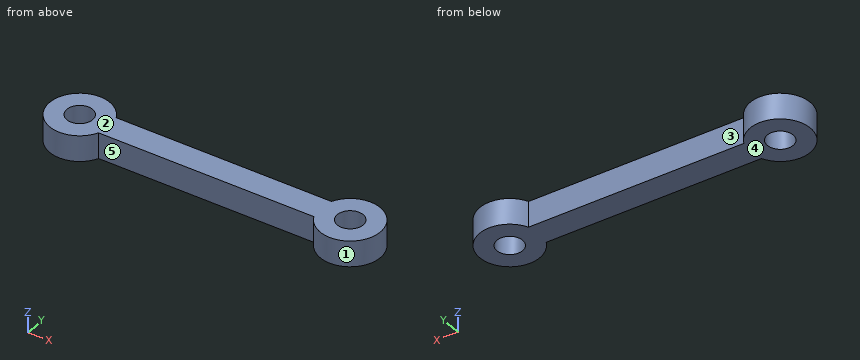
Autodesk Fusion 360 part; units mm, degrees
sketch "Sketch1" plane through (0, 0, 0) normal (0, 0, 1) x (1, 0, 0)
  circle A0 centre (-30.1129, -14.4636) radius 3.5
  circle A1 centre (-30.1129, -14.4636) radius 1.5
  line L0 (-30.1129, -14.4636) -> (0.8871, -14.4636)
  line L1 (-14.6129, -4.9636) -> (-14.6129, -23.9636) construction
  circle A2 centre (0.8871, -14.4636) radius 3.5
  circle A3 centre (0.8871, -14.4636) radius 1.5
  line L2 (-26.9506, -12.9636) -> (-2.2752, -12.9636)
  line L3 (-26.9506, -15.9636) -> (-2.2752, -15.9636)
  point P0 (0.8871, -14.4636)
  dimension "d1" = 7
  dimension "d2" = 3
  dimension "d3" = 31
  dimension "d4" = 1.5
extrude "Extrude1" add sketch "Sketch1" along normal blind 3
Design review of the part built by this model. Coordinates are the model's own, in mm. Face numbers are marked on the shaded views. A direction names the side the tool comes from. Coordinates: 2 decimals unless noted, no trailing zeros. Loops run counter-clockwise (first coordinate to the right, second up) from the corner with the lowest first, then second, coordinate; pieces in that order, holes last. Notation, with made-up numbers: (11, 40.25) -> (42, 40.25) arc R19 ccw to (42, 68.25) -> close; hole circle Ø8 at (10, -14.75). An arc over 180 degrees is marked (long way). Answer as a JSON object with one key per item and string values.
Q1. Take a section at C-C on z = 1.15. Give the boundary of the cut face in (x, y), plus the area to 3 significant figures.
Answer block:
{"outline": "(-26.95, -15.96) -> (-2.28, -15.96) arc R3.5 ccw (long way) to (-2.28, -12.96) -> (-26.95, -12.96) arc R3.5 ccw (long way) to start; hole circle Ø3 at (-30.11, -14.46); hole circle Ø3 at (0.89, -14.46)", "area": "135 mm^2"}
Q2. Take a section at D-D on x = -14. Give the boundary of the cut face in (y, z).
Answer block:
{"outline": "(-15.96, 0) -> (-12.96, 0) -> (-12.96, 3) -> (-15.96, 3) -> close"}
Q3. To check wall thickness, follow L1, parallel to X at y = -15, z = 0.75; L2, parallel to X at y = -14.75, z = 1.8; L3, parallel to Y at x = -13, z = 1.3. State the ranges of each line that lie inside material, in increasing order.
Answer block:
{"L1": "x = -33.57 to -31.51, -28.71 to -0.51, 2.29 to 4.35", "L2": "x = -33.6 to -31.59, -28.64 to -0.59, 2.36 to 4.38", "L3": "y = -15.96 to -12.96"}
Q4. The part is to be moulded in two halves that separate along X. For the marked faces 1 and 2, say which applies: +X half, -X half, draft (parallel to the pull), parting line (faces both ways), or undercut.
Answer block:
{"face 1": "undercut", "face 2": "draft"}
Q5. Tool access review of the marked faces 3, 4 and 5: name each direction out of +Z, -Z, +X, -X, +Y, -Y from which nothing blocks a thin tool from reaching the whole face with its end or side.
Answer block:
{"face 3": "+Z, -Z, +Y", "face 4": "-Z, +X, -X, +Y, -Y", "face 5": "+Z, -Z, -Y"}
Q6. Take a section at A-A on y = -17. Give the boundary of the cut face in (x, z).
Answer block:
{"outline": "(-32.52, 0) -> (-27.7, 0) -> (-27.7, 3) -> (-32.52, 3) -> close; (-1.52, 0) -> (3.3, 0) -> (3.3, 3) -> (-1.52, 3) -> close"}
Q7. Clearance check with a flat-ended pin moving along its axis: pin 1 Ø1.5 at (y, z) = (-14, 1) entering from -X. State where the tip first meets the part, or that it passes through.
Answer block:
{"pin 1": "stops at x = -33.61"}
Q8. Take a section at B-B on y = -14. Give the boundary of the cut face in (x, z), plus the area to 3 significant figures.
Answer block:
{"outline": "(-33.58, 0) -> (-31.54, 0) -> (-31.54, 3) -> (-33.58, 3) -> close; (-28.69, 0) -> (-0.54, 0) -> (-0.54, 3) -> (-28.69, 3) -> close; (2.31, 0) -> (4.36, 0) -> (4.36, 3) -> (2.31, 3) -> close", "area": "96.7 mm^2"}
